```python
from build123d import *

# Parameters (mm, degrees)
SKETCH1_W           = 33.02
SKETCH1_H           = 20.32
BOSS_EXTRUDE1_DEPTH = 6.35
SKETCH2_W           = 20.32
SKETCH2_H           = 33.02
BOSS_EXTRUDE2_DEPTH = 6.35
BOSS_EXTRUDE3_DEPTH = 33.02
SKETCH6_R           = 6.35
CUT_EXTRUDE1_DEPTH  = 61.787777554
SKETCH7_R           = 6.35
CUT_EXTRUDE2_DEPTH  = 58.065270644


with BuildPart() as part:
    # Sketch1 → Boss-Extrude1 (new body)
    with BuildSketch(Plane(origin=(0, 0, 0), x_dir=(0, 0, -1), z_dir=(1, 0, 0))):
        Rectangle(SKETCH1_W, SKETCH1_H)
    extrude(amount=BOSS_EXTRUDE1_DEPTH)

    # Sketch5 → #6-32 Tapped Hole1 (revolve, cut)
    with BuildSketch(Plane(origin=(3.175, 0, -16.51), x_dir=(0, 1, 0), z_dir=(1, 0, 0))):
        Polygon((0, 0), (0, 9.44869403), (1.35255, 8.636), (1.35255, 0), align=None)
    revolve(axis=Axis((3.175, 0, -22.86), (0, 0, 1)), mode=Mode.SUBTRACT)

    # Sketch5 at point 2 (carried to point 2, square into its face) → #6-32 Tapped Hole1 at 2 (revolve, cut)
    with BuildSketch(Plane(origin=(3.175, 10.16, 0), x_dir=(0, 0, 1), z_dir=(1, 0, 0))):
        Polygon((0, 0), (0, 9.44869403), (1.35255, 8.636), (1.35255, 0), align=None)
    revolve(axis=Axis((3.175, 16.51, 0), (0, -1, 0)), mode=Mode.SUBTRACT)

    # Sketch5 at point 7 (carried to point 7, square into its face) → #6-32 Tapped Hole1 at 7 (revolve, cut)
    with BuildSketch(Plane(origin=(3.175, 0, 16.51), x_dir=(0, 1, 0), z_dir=(-1, 0, 0))):
        Polygon((0, 0), (0, 9.44869403), (1.35255, 8.636), (1.35255, 0), align=None)
    revolve(axis=Axis((3.175, 0, 22.86), (0, 0, -1)), mode=Mode.SUBTRACT)

    # Sketch5 at point 8 (carried to point 8, square into its face) → #6-32 Tapped Hole1 at 8 (revolve, cut)
    with BuildSketch(Plane(origin=(3.175, -10.16, 0), x_dir=(0, 0, -1), z_dir=(1, 0, 0))):
        Polygon((0, 0), (0, 9.44869403), (1.35255, 8.636), (1.35255, 0), align=None)
    revolve(axis=Axis((3.175, -16.51, 0), (0, 1, 0)), mode=Mode.SUBTRACT)



with BuildPart() as body_2:
    # Sketch2 → Boss-Extrude2 (new body)
    with BuildSketch(Plane(origin=(0, 10.16, 0), x_dir=(1, 0, 0), z_dir=(0, 1, 0))):
        with Locations((41.91, 0)):
            Rectangle(SKETCH2_W, SKETCH2_H)
    extrude(amount=BOSS_EXTRUDE2_DEPTH)

    # Sketch5 at point 3 (carried to point 3, square into its face) → #6-32 Tapped Hole1 at 3 (revolve, cut)
    with BuildSketch(Plane(origin=(31.75, 13.335, 0), x_dir=(0, 1, 0), z_dir=(0, 0, -1))):
        Polygon((0, 0), (0, 9.44869403), (1.35255, 8.636), (1.35255, 0), align=None)
    revolve(axis=Axis((25.4, 13.335, 0), (1, 0, 0)), mode=Mode.SUBTRACT)

    # Sketch5 at point 4 (carried to point 4, square into its face) → #6-32 Tapped Hole1 at 4 (revolve, cut)
    with BuildSketch(Plane(origin=(41.91, 13.335, -16.51), x_dir=(0, 1, 0), z_dir=(1, 0, 0))):
        Polygon((0, 0), (0, 9.44869403), (1.35255, 8.636), (1.35255, 0), align=None)
    revolve(axis=Axis((41.91, 13.335, -22.86), (0, 0, 1)), mode=Mode.SUBTRACT)

    # Sketch5 at point 5 (carried to point 5, square into its face) → #6-32 Tapped Hole1 at 5 (revolve, cut)
    with BuildSketch(Plane(origin=(41.91, 13.335, 16.51), x_dir=(0, 1, 0), z_dir=(-1, 0, 0))):
        Polygon((0, 0), (0, 9.44869403), (1.35255, 8.636), (1.35255, 0), align=None)
    revolve(axis=Axis((41.91, 13.335, 22.86), (0, 0, -1)), mode=Mode.SUBTRACT)

    # Sketch5 at point 6 (carried to point 6, square into its face) → #6-32 Tapped Hole1 at 6 (revolve, cut)
    with BuildSketch(Plane(origin=(52.07, 13.335, 0), x_dir=(0, 1, 0), z_dir=(0, 0, 1))):
        Polygon((0, 0), (0, 9.44869403), (1.35255, 8.636), (1.35255, 0), align=None)
    revolve(axis=Axis((58.42, 13.335, 0), (-1, 0, 0)), mode=Mode.SUBTRACT)


with BuildPart() as part_1:
    add(part.part)

    add(body_2.part)  # Boss-Extrude3 merges body 2
    # Sketch4 → Boss-Extrude3 (add, through all)
    with BuildSketch(Plane.XY.offset(-16.51)):
        Polygon((52.07, 10.16), (52.07, 3.81), (12.7, -10.16), (6.35, -10.16), (6.35, 10.16), align=None)
    extrude(amount=BOSS_EXTRUDE3_DEPTH)

    # Sketch6 → Cut-Extrude1 (cut, through all)
    with BuildSketch(Plane(origin=(0, 16.51, 0), x_dir=(1, 0, 0), z_dir=(0, 1, 0))):
        with Locations(Location((41.91, 0, 0), (0, 0, 270))):
            Circle(SKETCH6_R)
    extrude(amount=-CUT_EXTRUDE1_DEPTH, mode=Mode.SUBTRACT)

    # Sketch7 → Cut-Extrude2 (cut, through all)
    with BuildSketch(Plane.ZY):
        Circle(SKETCH7_R)
    extrude(amount=-CUT_EXTRUDE2_DEPTH, mode=Mode.SUBTRACT)


solid = part_1.part
```
Check sheet for the modelled part. Datum: model origin and axes. Units: mm. A direction names the side the tool comes from. Give positions to 0.01 mm unless a question says otherwise; leave off trailing zeros. Order: outer loops, then holes, each group sorted by start corner. A loop starts at its lowest first (then second) coordinate and runs counter-clockwise, first axis right, second up. Notation, with made-up numbers: M 48,-38.75 L 60,-38.75 A22 cw 60,-10.75 Z; hole C 13.5,69 d10. An arc over 180 degrees is marked long. Answer in a Markdown table with one row per item.
1) Access from +Z, -Z, +X, -X, +Y, -Y to the whole of each face (thin tool, end or side, straight path). Record for faces 5 (the flat face through (31.75, 15, 0)), 6 (the flat face through (6, -10.16, 0)), 7 (the cylindrical face through (4.495, -0.293, -12.252)).
Filled sheet:
| item | result |
|---|---|
| face 5 | +Z, -Z, -X, +Y |
| face 6 | +Z, -Z, +X, -X, -Y |
| face 7 | -Z |
2) Thickness scan on L1, parallel to Z at x = 31.5, y = -0.25; L2, parallel to Y at x = 24, z = 0; L3, parallel to Z at x = 36, y = -1.75. Record the ranges inside material, lowest first. Write a range as [from, to].
Filled sheet:
| item | result |
|---|---|
| L1 | z = [-16.51, -6.35], [6.35, 16.51] |
| L2 | y = [6.35, 10.16] |
| L3 | z = [-16.51, -6.1], [6.1, 16.51] |
3) Cross-section at A-A, the plane x = 12. Enter the section's corners in (y, z), plus the area to 3 significant figures.
Filled sheet:
| item | result |
|---|---|
| outline | M -10.16,-16.51 L 10.16,-16.51 L 10.16,16.51 L -10.16,16.51 Z; hole C 0,0 d12.7 |
| area | 544 mm2 |
4) Gauge pin test, flat ends, axial feed: P1, Ø1, axis at x = 21, z = -5.5, coming from the -Y side; P2, Ø1.6, axis at x = 41.91, y = 13.335, coming from the -Z side; P3, Ø10, axis at y = 0, z = 0, coming from the +X side; P4, Ø9.5, axis at x = 21.5, z = 4, coming from the +Y side. Record the tip position at first contact, or that the pin passes through.
Filled sheet:
| item | result |
|---|---|
| P1 | stops at y = -7.39 |
| P2 | stops at z = -7.54 |
| P3 | passes through |
| P4 | stops at y = 10.16 |
5) Cross-section at C-C, the plane z = 0. Count the separate pieces of the cut face and the enclosed holes in it, plus the area to 3 significant figures.
Filled sheet:
| item | result |
|---|---|
| separate pieces | 7 |
| enclosed holes | 0 |
| area | 226 mm2 |
6) Cross-section at D-D, the plane z = -10. Enter the section's corners in (x, y) (3 decimals).
Filled sheet:
| item | result |
|---|---|
| outline | M 0,-10.16 L 12.7,-10.16 L 52.07,3.81 L 52.07,16.51 L 31.75,16.51 L 31.75,10.16 L 0,10.16 Z; hole C 3.175,0 d2.705; hole C 41.91,13.335 d2.705 |
7) Cross-section at B-B, the plane y = -8.25. Enter the section's corners in (x, z) (3 decimals).
Filled sheet:
| item | result |
|---|---|
| outline | M 0,-16.51 L 18.083,-16.51 L 18.083,16.51 L 0,16.51 Z; hole C 3.175,0 d2.705 |
8) Release check for a two-part mould opening along Z. For faces 1 (the cylindrical face through (33.7, 11.984, 0.059)), 2 (the flat face through (49, 16.51, 0)), 3 (the conical face through (2.95, -0.05, 7.2)), 4 (the conical face through (41.712, 13.461, -7.202)) record: +Z half, -Z half, draft (parallel to the pull), parting line (faces both ways), or undercut.
Filled sheet:
| item | result |
|---|---|
| face 1 | undercut |
| face 2 | draft |
| face 3 | +Z half |
| face 4 | -Z half |
